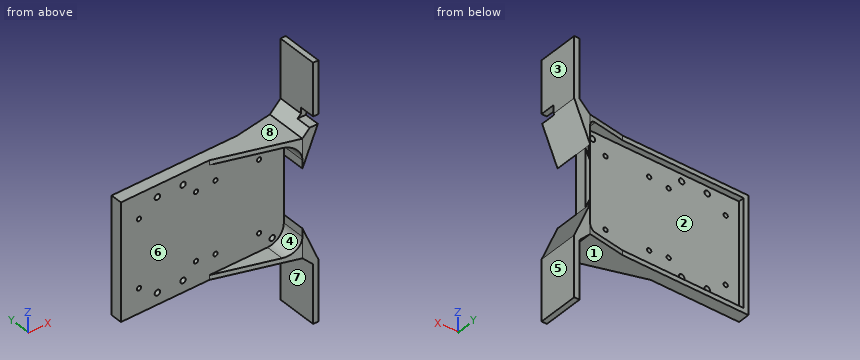
from build123d import *

# Parameters (mm, degrees)
SKETCH1_W                = 140
SKETCH1_H                = 100
BOSS_EXTRUDE1_DEPTH      = 10
SKETCH2_W                = 132
SKETCH2_H                = 92
CUT_EXTRUDE1_DEPTH       = 5
CUT_EXTRUDE2_REACH       = 88.168
SKETCH6_R                = 2.35
CUT_EXTRUDE3_REACH       = 88.168
SKETCH9_R                = 1.85
BOSS_EXTRUDE2_DEPTH      = 15
BOSS_EXTRUDE2_DEPTH_BACK = 20
BOSS_EXTRUDE3_DEPTH      = 4
FILLET3_R                = 5
FILLET4_R                = 5
FILLET5_R                = 5
FILLET6_R                = 5
FILLET7_R                = 14
CUT_EXTRUDE4_REACH       = 191.59
SKETCH13_W               = 8
SKETCH13_H               = 13


with BuildPart() as part:
    # Sketch1 → Boss-Extrude1 (new body)
    with BuildSketch(Plane(origin=(0, 0, 0), x_dir=(1, 0, 0), z_dir=(0, 1, 0))):
        Rectangle(SKETCH1_W, SKETCH1_H)
    extrude(amount=BOSS_EXTRUDE1_DEPTH)

    # Sketch2 → Cut-Extrude1 (cut)
    with BuildSketch(Plane(origin=(0, 10, 0), x_dir=(1, 0, 0), z_dir=(0, 1, 0))):
        Rectangle(SKETCH2_W, SKETCH2_H)
    extrude(amount=-CUT_EXTRUDE1_DEPTH, mode=Mode.SUBTRACT)

    # Sketch6 → Cut-Extrude2 (cut, up to next)
    with BuildSketch(Plane(origin=(0, 5, 0), x_dir=(1, 0, 0), z_dir=(0, 1, 0)), mode=Mode.PRIVATE) as cut_extrude2_sk1:
        with Locations(Location((60, 40, 0), (0, 0, 270))):
            Circle(SKETCH6_R)
    cut_extrude2_tool1 = extrude(cut_extrude2_sk1.sketch, amount=-CUT_EXTRUDE2_REACH, mode=Mode.PRIVATE) & part.part
    # Sketch6 → Cut-Extrude2 (cut, up to next)
    with BuildSketch(Plane(origin=(0, 5, 0), x_dir=(1, 0, 0), z_dir=(0, 1, 0)), mode=Mode.PRIVATE) as cut_extrude2_sk2:
        with Locations(Location((60, -40, 0), (0, 0, 270))):
            Circle(SKETCH6_R)
    cut_extrude2_tool2 = extrude(cut_extrude2_sk2.sketch, amount=-CUT_EXTRUDE2_REACH, mode=Mode.PRIVATE) & part.part
    # Sketch6 → Cut-Extrude2 (cut, up to next)
    with BuildSketch(Plane(origin=(0, 5, 0), x_dir=(1, 0, 0), z_dir=(0, 1, 0)), mode=Mode.PRIVATE) as cut_extrude2_sk3:
        with Locations(Location((-16.641543992, -40, 0), (0, 0, 270))):
            Circle(SKETCH6_R)
    cut_extrude2_tool3 = extrude(cut_extrude2_sk3.sketch, amount=-CUT_EXTRUDE2_REACH, mode=Mode.PRIVATE) & part.part
    # Sketch6 → Cut-Extrude2 (cut, up to next)
    with BuildSketch(Plane(origin=(0, 5, 0), x_dir=(1, 0, 0), z_dir=(0, 1, 0)), mode=Mode.PRIVATE) as cut_extrude2_sk4:
        with Locations(Location((-16.641543992, 40, 0), (0, 0, 270))):
            Circle(SKETCH6_R)
    cut_extrude2_tool4 = extrude(cut_extrude2_sk4.sketch, amount=-CUT_EXTRUDE2_REACH, mode=Mode.PRIVATE) & part.part
    # Sketch6 → Cut-Extrude2 (cut, up to next)
    with BuildSketch(Plane(origin=(0, 5, 0), x_dir=(1, 0, 0), z_dir=(0, 1, 0)), mode=Mode.PRIVATE) as cut_extrude2_sk5:
        with Locations(Location((-38.674837349, -40, 0), (0, 0, 270))):
            Circle(SKETCH6_R)
    cut_extrude2_tool5 = extrude(cut_extrude2_sk5.sketch, amount=-CUT_EXTRUDE2_REACH, mode=Mode.PRIVATE) & part.part
    # Sketch6 → Cut-Extrude2 (cut, up to next)
    with BuildSketch(Plane(origin=(0, 5, 0), x_dir=(1, 0, 0), z_dir=(0, 1, 0)), mode=Mode.PRIVATE) as cut_extrude2_sk6:
        with Locations(Location((-38.674837349, 40, 0), (0, 0, 270))):
            Circle(SKETCH6_R)
    cut_extrude2_tool6 = extrude(cut_extrude2_sk6.sketch, amount=-CUT_EXTRUDE2_REACH, mode=Mode.PRIVATE) & part.part
    add(cut_extrude2_tool1.solids().sort_by_distance((60, 5, -40))[0], mode=Mode.SUBTRACT)
    add(cut_extrude2_tool2.solids().sort_by_distance((60, 5, 40))[0], mode=Mode.SUBTRACT)
    add(cut_extrude2_tool3.solids().sort_by_distance((-16.641544, 5, 40))[0], mode=Mode.SUBTRACT)
    add(cut_extrude2_tool4.solids().sort_by_distance((-16.641544, 5, -40))[0], mode=Mode.SUBTRACT)
    add(cut_extrude2_tool5.solids().sort_by_distance((-38.674837, 5, 40))[0], mode=Mode.SUBTRACT)
    add(cut_extrude2_tool6.solids().sort_by_distance((-38.674837, 5, -40))[0], mode=Mode.SUBTRACT)

    # Sketch9 → Cut-Extrude3 (cut, up to next)
    with BuildSketch(Plane(origin=(0, 5, 0), x_dir=(1, 0, 0), z_dir=(0, 1, 0)), mode=Mode.PRIVATE) as cut_extrude3_sk1:
        with Locations(Location((-54.5, 29, 0), (0, 0, 270))):
            Circle(SKETCH9_R)
    cut_extrude3_tool1 = extrude(cut_extrude3_sk1.sketch, amount=-CUT_EXTRUDE3_REACH, mode=Mode.PRIVATE) & part.part
    # Sketch9 → Cut-Extrude3 (cut, up to next)
    with BuildSketch(Plane(origin=(0, 5, 0), x_dir=(1, 0, 0), z_dir=(0, 1, 0)), mode=Mode.PRIVATE) as cut_extrude3_sk2:
        with Locations(Location((-5.5, 29, 0), (0, 0, 270))):
            Circle(SKETCH9_R)
    cut_extrude3_tool2 = extrude(cut_extrude3_sk2.sketch, amount=-CUT_EXTRUDE3_REACH, mode=Mode.PRIVATE) & part.part
    # Sketch9 → Cut-Extrude3 (cut, up to next)
    with BuildSketch(Plane(origin=(0, 5, 0), x_dir=(1, 0, 0), z_dir=(0, 1, 0)), mode=Mode.PRIVATE) as cut_extrude3_sk3:
        with Locations(Location((-54.5, -29, 0), (0, 0, 270))):
            Circle(SKETCH9_R)
    cut_extrude3_tool3 = extrude(cut_extrude3_sk3.sketch, amount=-CUT_EXTRUDE3_REACH, mode=Mode.PRIVATE) & part.part
    # Sketch9 → Cut-Extrude3 (cut, up to next)
    with BuildSketch(Plane(origin=(0, 5, 0), x_dir=(1, 0, 0), z_dir=(0, 1, 0)), mode=Mode.PRIVATE) as cut_extrude3_sk4:
        with Locations(Location((-5.5, -29, 0), (0, 0, 270))):
            Circle(SKETCH9_R)
    cut_extrude3_tool4 = extrude(cut_extrude3_sk4.sketch, amount=-CUT_EXTRUDE3_REACH, mode=Mode.PRIVATE) & part.part
    # Sketch9 → Cut-Extrude3 (cut, up to next)
    with BuildSketch(Plane(origin=(0, 5, 0), x_dir=(1, 0, 0), z_dir=(0, 1, 0)), mode=Mode.PRIVATE) as cut_extrude3_sk5:
        with Locations(Location((11.25, 30.75, 0), (0, 0, 270))):
            Circle(SKETCH9_R)
    cut_extrude3_tool5 = extrude(cut_extrude3_sk5.sketch, amount=-CUT_EXTRUDE3_REACH, mode=Mode.PRIVATE) & part.part
    # Sketch9 → Cut-Extrude3 (cut, up to next)
    with BuildSketch(Plane(origin=(0, 5, 0), x_dir=(1, 0, 0), z_dir=(0, 1, 0)), mode=Mode.PRIVATE) as cut_extrude3_sk6:
        with Locations(Location((48.75, 30.75, 0), (0, 0, 270))):
            Circle(SKETCH9_R)
    cut_extrude3_tool6 = extrude(cut_extrude3_sk6.sketch, amount=-CUT_EXTRUDE3_REACH, mode=Mode.PRIVATE) & part.part
    # Sketch9 → Cut-Extrude3 (cut, up to next)
    with BuildSketch(Plane(origin=(0, 5, 0), x_dir=(1, 0, 0), z_dir=(0, 1, 0)), mode=Mode.PRIVATE) as cut_extrude3_sk7:
        with Locations(Location((48.75, -30.75, 0), (0, 0, 270))):
            Circle(SKETCH9_R)
    cut_extrude3_tool7 = extrude(cut_extrude3_sk7.sketch, amount=-CUT_EXTRUDE3_REACH, mode=Mode.PRIVATE) & part.part
    # Sketch9 → Cut-Extrude3 (cut, up to next)
    with BuildSketch(Plane(origin=(0, 5, 0), x_dir=(1, 0, 0), z_dir=(0, 1, 0)), mode=Mode.PRIVATE) as cut_extrude3_sk8:
        with Locations(Location((11.25, -30.75, 0), (0, 0, 270))):
            Circle(SKETCH9_R)
    cut_extrude3_tool8 = extrude(cut_extrude3_sk8.sketch, amount=-CUT_EXTRUDE3_REACH, mode=Mode.PRIVATE) & part.part
    add(cut_extrude3_tool1.solids().sort_by_distance((-54.5, 5, -29))[0], mode=Mode.SUBTRACT)
    add(cut_extrude3_tool2.solids().sort_by_distance((-5.5, 5, -29))[0], mode=Mode.SUBTRACT)
    add(cut_extrude3_tool3.solids().sort_by_distance((-54.5, 5, 29))[0], mode=Mode.SUBTRACT)
    add(cut_extrude3_tool4.solids().sort_by_distance((-5.5, 5, 29))[0], mode=Mode.SUBTRACT)
    add(cut_extrude3_tool5.solids().sort_by_distance((11.25, 5, -30.75))[0], mode=Mode.SUBTRACT)
    add(cut_extrude3_tool6.solids().sort_by_distance((48.75, 5, -30.75))[0], mode=Mode.SUBTRACT)
    add(cut_extrude3_tool7.solids().sort_by_distance((48.75, 5, 30.75))[0], mode=Mode.SUBTRACT)
    add(cut_extrude3_tool8.solids().sort_by_distance((11.25, 5, 30.75))[0], mode=Mode.SUBTRACT)

    # Sketch11 → Boss-Extrude2 (add, two sides: drawn at the far end of the back side and taken through both)
    with BuildSketch(Plane(origin=(0, 0, 0), x_dir=(1, 0, 0), z_dir=(0, 1, 0)).offset(-BOSS_EXTRUDE2_DEPTH_BACK)):
        Polygon((70, 50), (79.192388155, 59.192388155), (79.192388155, 109.192388155), (83.692388155, 109.192388155), (83.692388155, 57.25724503), (70, 25), align=None)
        Polygon((70, -25), (70, -50), (79.192388155, -59.192388155), (79.192388155, -109.192388155), (83.692388155, -109.192388155), (83.692388155, -57.25724503), align=None)
    extrude(amount=BOSS_EXTRUDE2_DEPTH + BOSS_EXTRUDE2_DEPTH_BACK)

    # Sketch12 → Boss-Extrude3 (add)
    with BuildSketch(Plane(origin=(0, 0, -50), x_dir=(-1, 0, 0), z_dir=(0, 0, -1))):
        Polygon((-70, 15), (-38, 10), (-70, 10), align=None)
        Polygon((-70, -20), (-70, 0), (-6, 0), align=None)
    boss_extrude3 = extrude(amount=-BOSS_EXTRUDE3_DEPTH)

    # Fillet3
    # the kernel refuses this fillet: 5 mm, written as the material it adds along each edge
    with BuildSketch(Plane(origin=(70, 10, -58.247448714), x_dir=(0, 1, 0), z_dir=(0, 0, 1))) as fillet3_piece_1_section:
        with BuildLine():
            CenterArc((4.898979486, 5), FILLET3_R, 191.536959033, 78.463040967)
            Line((0, 4), (0, 0))
            Line((0, 0), (4.898979486, 0))
        make_face()
    fillet3_piece_1 = extrude(amount=45.494897428, mode=Mode.PRIVATE)
    fillet3_piece_1 = split(fillet3_piece_1, bisect_by=Plane(origin=(81.95810656, 10, -53.17153363), z_dir=(-0.9205048534524429, 0, -0.3907311284892677)), keep=Keep.TOP, mode=Mode.PRIVATE)
    fillet3_piece_1 = split(fillet3_piece_1, bisect_by=Plane(origin=(74.123724357, 10, -54.123724357), z_dir=(0.7071067811865478, 0, 0.7071067811865472)), keep=Keep.TOP, mode=Mode.PRIVATE)
    add(fillet3_piece_1)

    # Fillet4
    # the kernel refuses this fillet: 5 mm, written as the material it adds along each edge
    with BuildSketch(Plane(origin=(70, 2.398979486, -46), x_dir=(0, 0, 1), z_dir=(0, 1, 0))) as fillet4_piece_1_section:
        with BuildLine():
            CenterArc((FILLET4_R, -FILLET4_R), FILLET4_R, 90, 90)
            Line((0, -FILLET4_R), (0, 0))
            Line((0, 0), (FILLET4_R, 0))
        make_face()
    fillet4_piece_1 = extrude(amount=25.101020514, mode=Mode.PRIVATE)
    fillet4_piece_1 = split(fillet4_piece_1, bisect_by=Plane(origin=(68.07801403, 14.699689692, -46), z_dir=(0.15437688027360966, -0.9880120337511015, 0)), keep=Keep.TOP, mode=Mode.PRIVATE)
    add(fillet4_piece_1)

    # Mirror6: Boss-Extrude3 across plane
    add(boss_extrude3.mirror(Plane.XY))

    # Fillet5
    # the kernel refuses this fillet: 5 mm, written as the material it adds along each edge
    with BuildSketch(Plane(origin=(70, 10, 12.752551286), x_dir=(-1.0, 1.5649703755111202e-12, 0), z_dir=(0, 0, 1))) as fillet5_piece_1_section:
        with BuildLine():
            CenterArc((5, -4.898979486), FILLET5_R, 101.536959033, 78.463040967)
            Line((0, -4.898979486), (0, 0))
            Line((0, 0), (4, 0))
        make_face()
    fillet5_piece_1 = extrude(amount=45.494897428, mode=Mode.PRIVATE)
    fillet5_piece_1 = split(fillet5_piece_1, bisect_by=Plane(origin=(51.376275643, 10, 31.376275643), z_dir=(0.7071067811865478, 0, -0.7071067811865472)), keep=Keep.TOP, mode=Mode.PRIVATE)
    fillet5_piece_1 = split(fillet5_piece_1, bisect_by=Plane(origin=(65.594961344, 10, 14.62237926), z_dir=(-0.9205048534524429, 0, 0.3907311284892677)), keep=Keep.TOP, mode=Mode.PRIVATE)
    add(fillet5_piece_1)

    # Fillet6
    # the kernel refuses this fillet: 5 mm, written as the material it adds along each edge
    with BuildSketch(Plane(origin=(70, 2.398979486, 46), x_dir=(-1, 0, 0), z_dir=(0, 1, 0))) as fillet6_piece_1_section:
        with BuildLine():
            CenterArc((FILLET6_R, -FILLET6_R), FILLET6_R, 90, 90)
            Line((0, -FILLET6_R), (0, 0))
            Line((0, 0), (FILLET6_R, 0))
        make_face()
    fillet6_piece_1 = extrude(amount=25.101020514, mode=Mode.PRIVATE)
    fillet6_piece_1 = split(fillet6_piece_1, bisect_by=Plane(origin=(68.07801403, 14.699689692, 46), z_dir=(0.15437688027360966, -0.9880120337511015, 0)), keep=Keep.TOP, mode=Mode.PRIVATE)
    add(fillet6_piece_1)

    # Fillet7
    fillet7_edges = [part.edges().sort_by_distance(p)[0] for p in [
        (70, -10, -46),
        (70, -10, 46),
    ]]
    fillet(fillet7_edges, radius=FILLET7_R)

    # Sketch13 → Cut-Extrude4 (cut, up to next)
    with BuildSketch(Plane(origin=(83.692388155, 0, 0), x_dir=(0, 0, -1), z_dir=(1, 0, 0)), mode=Mode.PRIVATE) as cut_extrude4_sk1:
        with Locations((-60.25724503, -13.5)):
            Rectangle(SKETCH13_W, SKETCH13_H)
    cut_extrude4_tool1 = extrude(cut_extrude4_sk1.sketch, amount=-CUT_EXTRUDE4_REACH, mode=Mode.PRIVATE) & part.part
    add(cut_extrude4_tool1.solids().sort_by_distance((83.692388, -13.5, 60.257245))[0], mode=Mode.SUBTRACT)


solid = part.part
Here's how the part is built. I have some questions about the finished solid (model axes, mm). Face numbers are marked on the shaded views. A direction names the side the tool comes from. Round coordinates to 2 decimals unless told otherwise and drop trailing zeros. Order: outer loops, then holes, each group sorted by start corner. A loop starts at its lowest first (then second) coordinate and runs counter-clockwise, first axis right, second up. Notation, with made-up numbers: (-37.5, 12) -> (-15.5, 12) arc R24 ccw to (-15.5, 29) -> close; hole circle Ø10 at (62.25, -5.75). An arc over 180 degrees is marked (long way). Return JSON: item names as keys, results as strings.
Q1. Which directions (+Z, -Z, +X, -X, +Y, -Y) give clear straight access to the entire face, cutting with the end or side of a thin tool? Please do the marked faces 5, 6, 7 and 8.
Filled sheet:
{"face 5": "+Z, -Z, +X, +Y, -Y", "face 6": "-X, -Y", "face 7": "-Z, -X, +Y, -Y", "face 8": "+Z, -X, +Y, -Y"}
Q2. If we section it at C-C on z = 90.5: List the corners of the cut face in (x, y) for me, plus the area to 4 significant figures.
Filled sheet:
{"outline": "(79.19, -20) -> (83.69, -20) -> (83.69, 15) -> (79.19, 15) -> close", "area": "157.5 mm^2"}
Q3. For pin 1 Ø4.5 at (x, y) = (-31.5, 9) entering from -Z; pin 2 Ø5.5 at (x, z) = (60, -40) entering from -Y; pin 3 Ø6 at (y, z) = (-7, -53.5) entering from +X, each with a flat end and sliding along its axis, tell me the tip position at first contact or that it passes through.
Filled sheet:
{"pin 1": "stops at z = -50", "pin 2": "stops at y = 0", "pin 3": "stops at x = 83.37"}
Q4. If we section it at A-A on y = -13: List the corners of the cut face in (x, z) for me.
Filled sheet:
{"outline": "(47.6, -50) -> (70, -50) -> (79.19, -59.19) -> (79.19, -109.19) -> (83.69, -109.19) -> (83.69, -57.26) -> (70, -25) -> (70, -32) arc R14 cw to (56, -46) -> (47.6, -46) -> close; (47.6, 46) -> (56, 46) arc R14 cw to (70, 32) -> (70, 25) -> (83.27, 56.26) -> (76.26, 56.26) -> (70, 50) -> (47.6, 50) -> close; (79.19, 64.26) -> (83.69, 64.26) -> (83.69, 109.19) -> (79.19, 109.19) -> close"}
Q5. If we section it at B-B on x = 60: Give the number of separate pieces and of enclosed holes in the cut face, plus the area to 3 significant figures.
Filled sheet:
{"separate pieces": "3", "enclosed holes": "0", "area": "675 mm^2"}
Q6. If we mould it in two halves opening along X, with no side actions, what happens to the marked faces 1, 2, 3 and 4? For each: released by +X, released by -X, zero draft, split by the parting line, or undercut.
Filled sheet:
{"face 1": "zero draft", "face 2": "undercut", "face 3": "released by +X", "face 4": "released by -X"}
Q7. I need wall thicknesses on line 1 along Z through (x, y) = (-57, 8); line 2 along X through (y, z) = (3, -40); line 3 along X through (y, z) = (-12, 97). Which ranges of each line are inside material? Lowest first, please. Write a range as from..to.
Filled sheet:
{"line 1": "z = -50..-46, 46..50", "line 2": "x = -70..-41.02, -36.32..-18.99, -14.29..57.65, 62.35..76.37", "line 3": "x = 79.19..83.69"}
